Build history of the part. All positions in model axes, mm. Face numbers are marked on the shaded views. Round coordinates to 2 decimals unless told otherwise and drop trailing zeros. Loops run counter-clockwise (first coordinate to the right, second up) from the corner with the lowest first, then second, coordinate; pieces in that order, holes last.
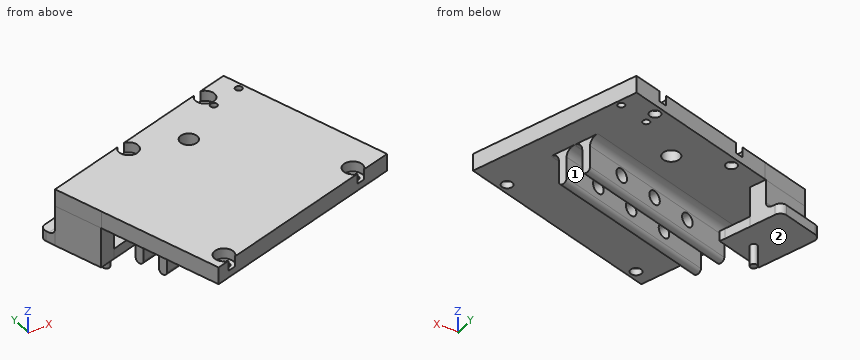
from build123d import *

# Parameters (mm, degrees)
BOSS_EXTRUDE1_DEPTH    = 5
BOSS_EXTRUDE3_DEPTH    = 11.75
BOSS_EXTRUDE5_DEPTH    = 3
FILLET1_R              = 2
BOSS_EXTRUDE6_DEPTH    = 10
SKETCH7_R              = 2
CUT_EXTRUDE1_DEPTH     = 96.909253568
BOSS_EXTRUDE8_DEPTH    = 3
FILLET4_R              = 2.5
FILLET5_R              = 1.25
CUT_EXTRUDE2_OUTLINE_R = 1.6
CUT_EXTRUDE2_DEPTH     = 5
SKETCH10_R             = 2.5
CUT_EXTRUDE3_DEPTH     = 110.504432364
SKETCH4_R              = 1
BOSS_EXTRUDE4_DEPTH    = 6
SKETCH12_R             = 2.8
CUT_EXTRUDE4_DEPTH     = 3
SKETCH9_R              = 1
CUT_EXTRUDE5_DEPTH     = 111.58128552


# Read off the part's stored shape, not the designer's step: Cut-Extrude2
# Some blends are built 0.0001 mm under size
with BuildPart() as part:
    # Sketch1 → Boss-Extrude1 (new body)
    with BuildSketch(Plane.XY):
        Polygon((21.227605409, -18.590227349), (16.764409011, -4.324804639), (31.175545422, 0.183980935), (77.940160264, 14.815139421), (93.586541992, -35.194367063), (32.410790739, -54.334311124), align=None)
    extrude(amount=BOSS_EXTRUDE1_DEPTH)

    # Sketch3 → Boss-Extrude3 (add)
    with BuildSketch(Plane(origin=(0, 0, 0), x_dir=(-1, 0, 0), z_dir=(0, 0, -1))):
        Polygon((-30.984669443, 0.124261921), (-32.477644799, -4.647637553), (-23.029283841, -7.603728757), (-25.939785869, -16.906376014), (-21.167886395, -18.39935137), (-16.764409011, -4.324804639), align=None)
    extrude(amount=BOSS_EXTRUDE3_DEPTH)

    # Sketch5 → Boss-Extrude5 (add)
    with BuildSketch(Plane(origin=(0, 0, -11.75), x_dir=(-1, 0, 0), z_dir=(0, 0, -1))):
        with BuildLine():
            Line((-30.984669443, 0.124261921), (-29.491694087, 4.896161395))
            Line((-29.491694087, 4.896161395), (-27.773810277, 4.358690267))
            Line((-27.773810277, 4.358690267), (-17.237837952, 1.062320107))
            ThreePointArc((-17.237837952, 1.062320107), (-16.072415286, 0.098650836), (-15.914708528, -1.405342859))
            Line((-15.914708528, -1.405342859), (-16.764409011, -4.324804639))
            Line((-16.764409011, -4.324804639), (-30.984669443, 0.124261921))
        make_face()
    extrude(amount=-BOSS_EXTRUDE5_DEPTH)

    # Fillet1
    fillet1_edges = [part.edges().sort_by_distance(p)[0] for p in [
        (23.874539227, -2.100271359, -8.75),
        (29.491694087, 4.896161395, -10.25),
    ]]
    fillet(fillet1_edges, radius=FILLET1_R)

    # Sketch6 → Boss-Extrude6 (add)
    with BuildSketch(Plane(origin=(0, 0, 0), x_dir=(-1, 0, 0), z_dir=(0, 0, -1))):
        Polygon((-77.85901424, -10.043127118), (-29.090201618, -25.301335253), (-28.34371394, -22.915385516), (-77.112526562, -7.657177381), align=None)
        Polygon((-79.351989595, -14.815026591), (-80.098477273, -17.200976328), (-31.329664652, -32.459184464), (-30.583176974, -30.073234727), align=None)
    extrude(amount=BOSS_EXTRUDE6_DEPTH)

    # Sketch7 → Cut-Extrude1 (cut, through all)
    with BuildSketch(Plane(origin=(9.057366854, -28.949469231, 0), x_dir=(0.9543798947428422, 0.29859507114257827, 0), z_dir=(-0.2985950711425783, 0.9543798947428423, 0))):
        with Locations(Location((46.758249559, 5, 0), (0, 0, 180))):
            Circle(SKETCH7_R)
        with Locations(Location((59.258249559, 5, 0), (0, 0, 180))):
            Circle(SKETCH7_R)
        with Locations(Location((34.258249559, 5, 0), (0, 0, 180))):
            Circle(SKETCH7_R)
    extrude(amount=-CUT_EXTRUDE1_DEPTH, mode=Mode.SUBTRACT)

    # Sketch11 → Boss-Extrude8 (add)
    with BuildSketch(Plane(origin=(0, 0, -11.75), x_dir=(-1, 0, 0), z_dir=(0, 0, -1))):
        Polygon((-32.477644799, -4.647637553), (-34.866405368, -12.282676711), (-35.388146827, -13.95028481), (-25.939785869, -16.906376014), (-23.029283841, -7.603728757), align=None)
    extrude(amount=-BOSS_EXTRUDE8_DEPTH)

    # Fillet4
    fillet4_edges = [part.edges().sort_by_distance(p)[0] for p in [
        (52.728120251, -15.286281449, 0),
        (53.474607929, -17.672231185, 0),
        (54.967583285, -22.444130659, 0),
        (55.714070963, -24.830080396, 0),
    ]]
    fillet(fillet4_edges, radius=FILLET4_R - 0.0001)  # a hair under: the kernel refuses the full size

    # Fillet5
    # the kernel refuses this fillet: 1.25 mm, written as the material it takes off along each edge
    with BuildSketch(Plane(origin=(83.080914444, -16.267866731, -10), x_dir=(0, 0, 1), z_dir=(-0.9543798947428422, -0.2985950711425782, 0)), Plane(origin=(27.600739803, -31.006344324, -10), x_dir=(0, 0, 1), z_dir=(0.9543798947428423, 0.2985950711425782, 0)), Plane(origin=(25.361276769, -23.848495114, -10), x_dir=(0, 0, 1), z_dir=(0.9543798947428422, 0.2985950711425783, 0)), Plane(origin=(80.841451411, -9.11001752, -10), x_dir=(0, 0, 1), z_dir=(-0.9543798947428422, -0.2985950711425783, 0))) as fillet5_piece_1:
        with BuildLine():
            CenterArc((FILLET5_R, FILLET5_R), FILLET5_R, 180, 90)
            Line((0, FILLET5_R), (0, 0))
            Line((0, 0), (FILLET5_R, 0))
        make_face()
    extrude(amount=57.35, mode=Mode.SUBTRACT)

    # Cut-Extrude2 outline → Cut-Extrude2 (cut)
    with BuildSketch(Plane.XY):
        with Locations((69.142848995, 9.443238973)):
            Circle(CUT_EXTRUDE2_OUTLINE_R)
        with Locations((36.436202535, -50.455386031)):
            Circle(CUT_EXTRUDE2_OUTLINE_R)
        with Locations((41.370394058, 0.754122403)):
            Circle(CUT_EXTRUDE2_OUTLINE_R)
        with Locations((83.296255367, -35.794368038)):
            Circle(CUT_EXTRUDE2_OUTLINE_R)
    extrude(amount=CUT_EXTRUDE2_DEPTH, mode=Mode.SUBTRACT)

    # Sketch10 → Cut-Extrude3 (cut, through all)
    with BuildSketch(Plane.XY.offset(5)):
        with Locations((56.022602403, -3.725145057)):
            Circle(SKETCH10_R)
    extrude(amount=-CUT_EXTRUDE3_DEPTH, mode=Mode.SUBTRACT)

    # Sketch4 → Boss-Extrude4 (add)
    with BuildSketch(Plane(origin=(0, 0, -11.75), x_dir=(-1, 0, 0), z_dir=(0, 0, -1))):
        with Locations((-27.213433721, -11.264996593)):
            Circle(SKETCH4_R)
    extrude(amount=BOSS_EXTRUDE4_DEPTH)

    # Sketch12 → Cut-Extrude4 (cut)
    with BuildSketch(Plane.XY.offset(5)):
        with Locations((69.142848995, 9.443238973)):
            Circle(SKETCH12_R)
        with Locations((41.370394058, 0.754122403)):
            Circle(SKETCH12_R)
        with Locations((36.436202535, -50.455386031)):
            Circle(SKETCH12_R)
        with Locations((83.296255367, -35.794368038)):
            Circle(SKETCH12_R)
    extrude(amount=-CUT_EXTRUDE4_DEPTH, mode=Mode.SUBTRACT)

    # Sketch9 → Cut-Extrude5 (cut, through all)
    with BuildSketch(Plane.XY.offset(5)):
        with Locations((78.168297598, 8.225179053)):
            Circle(SKETCH9_R)
        with Locations((69.101688598, 5.388525877)):
            Circle(SKETCH9_R)
    extrude(amount=-CUT_EXTRUDE5_DEPTH, mode=Mode.SUBTRACT)


solid = part.part
(1) Slice it at A-A on z = -15.5. List the corners of the cut face in (x, y) (3 decimals), plus the area to 3 significant figures.
Responses:
outline: circle Ø2 at (27.213, -11.265)
area: 3.14 mm2
(2) Slice it at B-B on y = -45. List the corners of the cut face in (x, z), plus the area to 3 significant figures.
Responses:
outline: (29.49, 0) - (62.25, 0) - (62.25, 5) - (29.49, 5) - close
area: 164 mm2
(3) Probe line 1 (Z direction, x = 80, y = 5.5); line 2 (X direction, y = -6, z = 1.5); line 3 (Y direction, x = 61, z = -0.5). List the from-to ranges inside material, lowest first.
Responses:
line 1: z = 0 to 5
line 2: x = 17.29 to 54.99, 57.06 to 84.45
line 3: y = -24.22 to -19.51, -16.37 to -11.65
(4) Pin check, flat tips, straight feed: P1, Ø5, axis at x = 83.3, y = -35.79, coming from the +Z side; P2, Ø1.5, axis at x = 43.5, z = -4, coming from the +Y side; P3, Ø2, axis at y = -3, z = 0.5, coming from the +X side. Stop position of each tip, or through.
Responses:
P1: stops at z = 2
P2: stops at y = -17.94
P3: stops at x = 83.83
(5) Pull direction X, two halves, no side cores. Call the marked faces 1 and 2: +X half, -X half, draft (parallel to the pull), parting line (faces both ways), or undercut.
Responses:
face 1: undercut
face 2: draft
